from build123d import *

# Parameters (mm, degrees)
F0_W     = 42
F0_H     = 25
F0_R     = 8.75
F1_DEPTH = 60
F0_R_2   = 5.1
F2_DEPTH = 35
F3_R     = 5.1
F4_DEPTH = 47.6


with BuildPart() as f1:
    # F0 (on Top) → F1 (new body)
    with BuildSketch(Plane.XY):
        with Locations((-2.65721, -27.237348)):
            Rectangle(F0_W, F0_H)
        with Locations((-11.65721, -27.237348)):
            Circle(F0_R, mode=Mode.SUBTRACT)
    extrude(amount=F1_DEPTH)

    # F0 (on Top) → F2 (join)
    with BuildSketch(Plane.XY):
        with Locations((-11.65721, -27.237348)):
            Circle(F0_R)
        with Locations((-11.65721, -27.237348)):
            Circle(F0_R_2, mode=Mode.SUBTRACT)
    extrude(amount=F2_DEPTH)

    # F3 (on face) → F4 (cut)
    with BuildSketch(Plane(origin=(0, -14.737348, 0), x_dir=(-1, 0, 0), z_dir=(0, 1, 0))):
        with Locations((-6.34279, 12)):
            Circle(F3_R)
    extrude(amount=-F4_DEPTH, mode=Mode.SUBTRACT)


solid = f1.part
Input: part model. Units: mm. Frame: model coordinates. Give positions to 0.01 mm unless a question says otherwise; leave off trailing zeros. Order: outer loops, then holes, each group sorted by start corner. A loop starts at its lowest first (then second) coordinate and runs counter-clockwise, first axis right, second up. Notation, with made-up numbers: (-19, 27.5) - (15, 27.5) arc R15 ccw to (15, 42.5) - close; hole circle Ø3 at (-2, 29.5). An arc over 180 degrees is marked (long way). Answer as a JSON object with one key per item and string values. Group by question number.
Q1. Line query: probe 1 along Z at (x, y) = (6.5, -36); probe 2 along Y at (x, z) = (-12, 48); probe 3 along X at (y, z) = (-27.25, 24). Output: solid intervals per line, ascending.
Q2. Cut plane A-A, the plane y = -29.75. Output: boundary loops of the cut face in (x, z).
Q3. Cut plane D-D, the plane y = -16.5. Output: boundary loops of the cut face in (x, z), then the cut area to 3 significant figures.
Q4. Mould query, pull axis X, two halves, no side actions, for faces 1 (the face through (-23.657, -27, 30)), 2 (the face through (-7.9, -31, 35)), 3 (the face through (-3, -14.737, 30)), 4 (the face through (-3.31, -24.61, 47.32)). Classes: pulls with the +X half, pulls with the -X half, needs draft (parallel to the pull), parting line crosses it, or undercut.
Q5. First-contact query: pin 1 Ø5 at (x, y) = (-13, -30) entering from +Z. Flat tip, straight axial feed; report the tip coordinate or a pass-through.
Q6. Cut plane C-C, the plane z = 9. Output: boundary loops of the cut face in (x, y).
Q7. Cut plane B-B, the plane x = -15. Output: boundary loops of the cut face in (y, z), then the cut area to 3 significant figures.
Results:
{
 "1": {"probe 1": "0 to 6.9, 17.1 to 60", "probe 2": "-39.74 to -35.98, -18.49 to -14.74", "probe 3": "-23.66 to -16.76, -6.56 to 18.34"},
 "2": {"outline": "(-23.66, 0) - (-16.1, 0) - (-16.1, 35) - (-20.04, 35) - (-20.04, 60) - (-23.66, 60) - close; (-7.22, 0) - (18.34, 0) - (18.34, 60) - (-3.28, 60) - (-3.28, 35) - (-7.22, 35) - close; hole circle Ø10.2 at (6.34, 12)"},
 "3": {"outline": "(-23.66, 0) - (18.34, 0) - (18.34, 60) - (-23.66, 60) - close; hole circle Ø10.2 at (6.34, 12)", "area": "2,440 mm^2"},
 "4": {"face 1": "pulls with the -X half", "face 2": "undercut", "face 3": "needs draft", "face 4": "undercut"},
 "5": {"pin 1": "z = 35"},
 "6": {"outline": "(-23.66, -39.74) - (2.22, -39.74) - (2.22, -14.74) - (-23.66, -14.74) - close; (10.47, -39.74) - (18.34, -39.74) - (18.34, -14.74) - (10.47, -14.74) - close; hole circle Ø10.2 at (-11.66, -27.24)"},
 "7": {"outline": "(-39.74, 0) - (-31.09, 0) - (-31.09, 35) - (-35.32, 35) - (-35.32, 60) - (-39.74, 60) - close; (-23.39, 0) - (-14.74, 0) - (-14.74, 60) - (-19.15, 60) - (-19.15, 35) - (-23.39, 35) - close", "area": "826 mm^2"}
}
